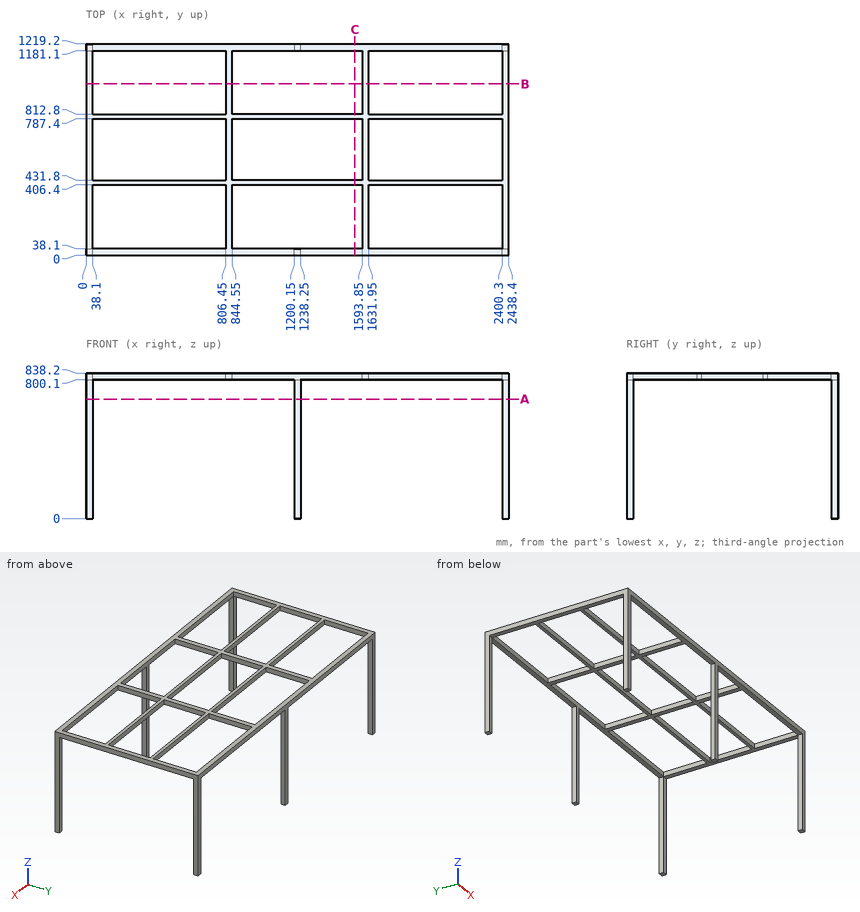
Can you work these out from the drawing? Everything is in mm from the part's minimum corner. Round coordinates to 2 decimals unless told otherwise and drop trailing zeros. Write each loop counter-clockwise with the first axis right and the second up, starting at its lowest first coordinate (ties: lowest second). Pieces come first, ordered by that corner, then holes.
1. Suppose I cut it at C-C (x = 1551.5). List the corners of the cut face in (y, z) for me.
2. Suppose I cut it at B-B (y = 989). List the corners of the cut face in (x, z) for me, and give its area (3 significant figures).
3. I need wall thicknesses on L1, parallel to Z at x = 187.5, y = 804. Which ranges of the line are inside material? Lowest first, please.
4. Suppose I cut it at A-A (z = 689.5). List the corners of the cut face in (x, y) for me.
5. Will this pin go through, and if not, where does the flat tip stop? pin 1 Ø19 at (y, z) = (1208.5, 425) entering from -X.
Answer sheet:
1. outline: (0, 800.1) - (38.1, 800.1) - (38.1, 838.2) - (0, 838.2) - close; (406.4, 800.1) - (431.8, 800.1) - (431.8, 838.2) - (406.4, 838.2) - close; (787.4, 800.1) - (812.8, 800.1) - (812.8, 838.2) - (787.4, 838.2) - close; (1181.1, 800.1) - (1219.2, 800.1) - (1219.2, 838.2) - (1181.1, 838.2) - close
2. outline: (0, 800.1) - (38.1, 800.1) - (38.1, 838.2) - (0, 838.2) - close; (806.45, 800.1) - (844.55, 800.1) - (844.55, 838.2) - (806.45, 838.2) - close; (1593.85, 800.1) - (1631.95, 800.1) - (1631.95, 838.2) - (1593.85, 838.2) - close; (2400.3, 800.1) - (2438.4, 800.1) - (2438.4, 838.2) - (2400.3, 838.2) - close
2. area: 5,810 mm2
3. L1: z = 800.1 to 838.2
4. outline: (0, 0) - (38.1, 0) - (38.1, 38.1) - (0, 38.1) - close; (0, 1181.1) - (38.1, 1181.1) - (38.1, 1219.2) - (0, 1219.2) - close; (1200.15, 0) - (1238.25, 0) - (1238.25, 38.1) - (1200.15, 38.1) - close; (1200.15, 1181.1) - (1238.25, 1181.1) - (1238.25, 1219.2) - (1200.15, 1219.2) - close; (2400.3, 0) - (2438.4, 0) - (2438.4, 38.1) - (2400.3, 38.1) - close; (2400.3, 1181.1) - (2438.4, 1181.1) - (2438.4, 1219.2) - (2400.3, 1219.2) - close
5. pin 1: stops at x = 0
